```python
from build123d import *

# Parameters (mm, degrees)
BOSS_EXTRUDE1_DEPTH = 7
FILLET1_R           = 2
SKETCH2_R           = 1.5
SKETCH2_R_2         = 1.1
BOSS_EXTRUDE2_DEPTH = 4
SKETCH3_R           = 1.5
SKETCH3_R_2         = 1.1
SKETCH3_W           = 4.5
SKETCH3_H           = 1.5
BOSS_EXTRUDE3_DEPTH = 4


with BuildPart() as part:
    # Sketch1 → Boss-Extrude1 (new body)
    with BuildSketch(Plane(origin=(0, 0, 0), x_dir=(1, 0, 0), z_dir=(0, 1, 0))):
        with BuildLine():
            Line((-10, 9), (10, 9))
            ThreePointArc((10, 9), (11.414213562, 8.414213562), (12, 7))
            Line((12, 7), (12, -7))
            ThreePointArc((12, -7), (11.414213562, -8.414213562), (10, -9))
            Line((10, -9), (-10, -9))
            ThreePointArc((-10, -9), (-11.414213562, -8.414213562), (-12, -7))
            Line((-12, -7), (-12, 7))
            ThreePointArc((-12, 7), (-11.414213562, 8.414213562), (-10, 9))
        make_face()
    extrude(amount=BOSS_EXTRUDE1_DEPTH)

    # Fillet1
    fillet1_edges = [part.edges().sort_by_distance(p)[0] for p in [
        (-12, 0, 0),
        (-11.414213562, 0, -8.414213562),
        (0, 0, -9),
        (11.414213562, 0, -8.414213562),
        (-11.414213562, 7, -8.414213562),
        (-12, 7, 0),
        (-11.414213562, 7, 8.414213562),
        (0, 7, 9),
        (11.414213562, 7, 8.414213562),
        (12, 7, 0),
        (11.414213562, 7, -8.414213562),
        (12, 0, 0),
        (0, 7, -9),
        (11.414213562, 0, 8.414213562),
        (0, 0, 9),
        (-11.414213562, 0, 8.414213562),
    ]]
    fillet(fillet1_edges, radius=FILLET1_R)

    # Sketch2 → Boss-Extrude2 (add)
    with BuildSketch(Plane.ZY.offset(12)):
        with Locations((-7, 3.5)):
            Circle(SKETCH2_R)
        with Locations((-7, 3.5)):
            Circle(SKETCH2_R_2, mode=Mode.SUBTRACT)
        with Locations((0, 3.5)):
            Circle(SKETCH2_R)
        with Locations((0, 3.5)):
            Circle(SKETCH2_R_2, mode=Mode.SUBTRACT)
        with Locations((7, 3.5)):
            Circle(SKETCH2_R)
        with Locations((7, 3.5)):
            Circle(SKETCH2_R_2, mode=Mode.SUBTRACT)
    extrude(amount=BOSS_EXTRUDE2_DEPTH)

    # Sketch3 → Boss-Extrude3 (add)
    with BuildSketch(Plane(origin=(12, 0, 0), x_dir=(0, 0, -1), z_dir=(1, 0, 0))):
        with Locations((-7, 3.5)):
            Circle(SKETCH3_R)
        with Locations((-7, 3.5)):
            Circle(SKETCH3_R_2, mode=Mode.SUBTRACT)
        with Locations((-2.6, 3.5)):
            Circle(SKETCH3_R)
        with Locations((-2.6, 3.5)):
            Circle(SKETCH3_R_2, mode=Mode.SUBTRACT)
        with Locations((4.379211167, 3.5)):
            Rectangle(SKETCH3_W, SKETCH3_H)
    extrude(amount=BOSS_EXTRUDE3_DEPTH)


solid = part.part
```
The listing builds one solid part. Answer for the finished solid, in the listing's coordinates (mm). A direction names the side the tool comes from. Give positions to 0.01 mm unless a question says otherwise; leave off trailing zeros. Loops run counter-clockwise (first coordinate to the right, second up) from the corner with the lowest first, then second, coordinate; pieces in that order, holes last. Notation, with made-up numbers: (52.25, 34.5) - (58.25, 34.5) arc R30 cw to (58.25, 67.5) - close; hole circle Ø2 at (61, -38.75). An arc over 180 degrees is marked (long way). Return JSON: item names as keys, results as strings. Group by question number.
1. Find section D-D (y = 3.5). State how many separate pieces and enclosed holes the cut face has, then the cut area to 3 significant figures.
2. Straight lines are drawn through the part: line 1 (Y direction, x = 13.45, z = 7); line 2 (X direction, y = 3.5, z = -5); line 3 (X direction, y = 3, z = -1.75). For each, find the intervals that lie inside material, in ascending order. Write a range as [from, to].
3. Determine the mould class of faces 1 (the cylindrical face through (-13.97, 4.43, 0.59)), 2 (the cylindrical face through (11.4, 3.48, -8.43)), 3 (the flat face through (0, 0, 0)) for opening direction Z: pulls with the +Z half, pulls with the -Z half, needs draft (parallel to the pull), parting line crosses it, or undercut.
4. Find section B-B (x = -9). Write down the section's boundary in (y, z), then the cut area to 3 significant figures.
5. Given pin 1 Ø0.5 at (y, z) = (4, -7.5) entering from +X; pin 2 Ø1.5 at (x, z) = (-12, 6.5) entering from +Y; pin 3 Ø3 at (x, z) = (14.5, -5) entering from +Y, each flat-ended and moving along its own axis, determine where each tip first touches the part or whether it passes through.
6. Find section A-A (x = 14). Write down the section's boundary in (y, z).
7. Find section C-C (z = 7.75). Write down the section's boundary in (x, y), then the cut area to 3 significant figures.
8. Which of the six approach directions +Z, -Z, +X, -X, +Y, -Y give full straight-line access (tool end or side, diameter ignored) to faces 4 (the flat face through (12, 3, 3)), 5 (the cylindrical face through (0.14, 6.4, -8.43))?
Verdict:
{
 "1": {"separate pieces": "4", "enclosed holes": "0", "area": "463 mm^2"},
 "2": {"line 1": "y = [2, 2.4], [4.6, 5]", "line 2": "x = [-12, 16]", "line 3": "x = [-12, 12]"},
 "3": {"face 1": "undercut", "face 2": "pulls with the -Z half", "face 3": "needs draft"},
 "4": {"outline": "(0, -7) arc R2 ccw to (2, -9) - (5, -9) arc R2 ccw to (7, -7) - (7, 7) arc R2 ccw to (5, 9) - (2, 9) arc R2 ccw to (0, 7) - close", "area": "123 mm^2"},
 "5": {"pin 1": "stops at x = 11.98", "pin 2": "stops at y = 6.56", "pin 3": "stops at y = 4.25"},
 "6": {"outline": "circle Ø3 at (3.5, 2.6); circle Ø3 at (3.5, 7); (2.75, -6.63) - (4.25, -6.63) - (4.25, -2.13) - (2.75, -2.13) - close; hole circle Ø2.2 at (3.5, 2.6); hole circle Ø2.2 at (3.5, 7)"},
 "7": {"outline": "(-16, 2.2) - (-12, 2.2) - (-12, 2.7) - (-16, 2.7) - close; (-16, 4.3) - (-12, 4.3) - (-12, 4.8) - (-16, 4.8) - close; (-11.85, 2) arc R1.85 ccw to (-10, 0.15) - (10, 0.15) arc R1.85 ccw to (11.85, 2) - (11.85, 5) arc R1.85 ccw to (10, 6.85) - (-10, 6.85) arc R1.85 ccw to (-11.85, 5) - close; (12, 2.2) - (16, 2.2) - (16, 2.7) - (12, 2.7) - close; (12, 4.3) - (16, 4.3) - (16, 4.8) - (12, 4.8) - close", "area": "164 mm^2"},
 "8": {"face 4": "+X", "face 5": "-Z, +X, -X, +Y"}
}
